Check sheet for the drawn part. Datum: minimum x, y, z corner. Units: mm. Round coordinates to 2 decimals unless told otherwise and drop trailing zeros. Write each loop counter-clockwise with the first axis right and the second up, starting at its lowest first coordinate (ties: lowest second). Pieces come first, ordered by that corner, then holes. Notation, with made-up numbers: (55.5, -14.75) -> (62.5, -14.75) arc R29 cw to (62.5, 24.25) -> close; hole circle Ø2 at (-1, 57.5). An arc over 180 degrees is marked (long way). One line per item, written item: value. Start each with the question number.
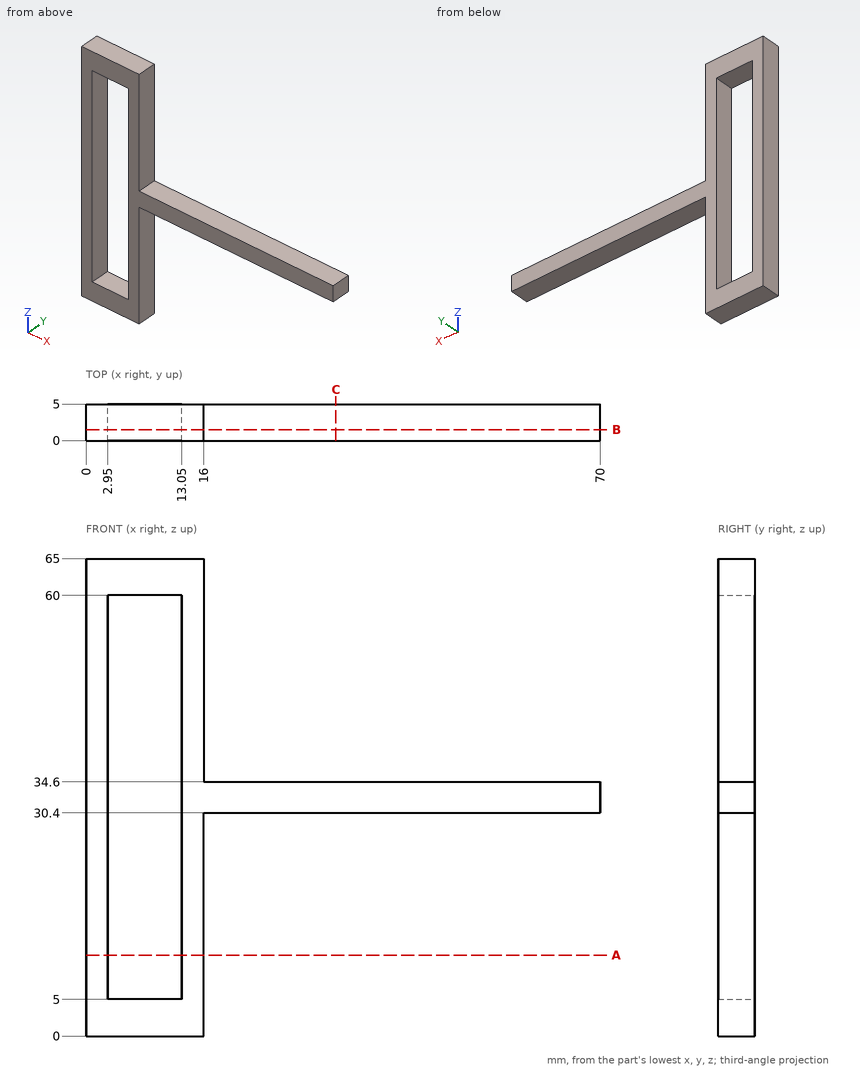
1. Cross-section at C-C (x = 34). Record the cut outline in (y, z), plus the area to 3 significant figures.
2. Cross-section at A-A (z = 11). Record the cut outline in (x, y), plus the area to 3 significant figures.
3. Cross-section at B-B (y = 1.5). Record the cut outline in (x, z), plus the area to 3 significant figures.
4. Depth check by flat-ended pin: pin 1 Ø2 at (x, y) = (47.5, 1.5) entering from -Z; pin 2 Ø2.5 at (x, y) = (48, 3.5) entering from +Z. Enter the tip coordinate at first touch or a pass-through.
5. Material ranges on probe 1 along X at (y, z) = (2.5, 29); probe 2 along Z at (x, y) = (7, 1.9); probe 3 along Z at (x, y) = (63.5, 3.85), recorded low to high.
Working result:
1. outline: (0, 30.4) -> (5, 30.4) -> (5, 34.6) -> (0, 34.6) -> close
1. area: 21.0 mm^2
2. outline: (0, 0) -> (2.95, 0) -> (2.95, 5) -> (0, 5) -> close; (13.05, 0) -> (16, 0) -> (16, 5) -> (13.05, 5) -> close
2. area: 29.5 mm^2
3. outline: (0, 0) -> (16, 0) -> (16, 30.4) -> (70, 30.4) -> (70, 34.6) -> (16, 34.6) -> (16, 65) -> (0, 65) -> close; hole (2.95, 5) -> (13.05, 5) -> (13.05, 60) -> (2.95, 60) -> close
3. area: 711 mm^2
4. pin 1: stops at z = 30.4
4. pin 2: stops at z = 34.6
5. probe 1: x = 0 to 2.95, 13.05 to 16
5. probe 2: z = 0 to 5, 60 to 65
5. probe 3: z = 30.4 to 34.6
